from build123d import *

# Parameters (mm, degrees)
F2_SIZE        = 0.5
F3_SIZE        = 0.5
F4_SIZE2       = 1.3397459622
F4_SIZE        = 5
F6_D           = 7
F7_D           = 7
F7_CBORE_D     = 11
F7_CBORE_DEPTH = 7.5
F9_D           = 6
F9_DEPTH       = 5
F9_TIP         = 1.8025818571


with BuildPart() as f1:
    # F0 (on Front) → F1 (revolve)
    with BuildSketch(Plane.XZ):
        Polygon((0, 32), (0, 0), (66, 0), (66, 6), (54.15, 6), (54.15, 32), align=None)
    revolve(axis=Axis((0, 0, 31.825657934), (0, 0, 1)))

    # F2
    f2_edges = [f1.edges().sort_by_distance(p)[0] for p in [
        (-66, 0, 6),
    ]]
    chamfer(f2_edges, length=F2_SIZE)

    # F3
    f3_edges = [f1.edges().sort_by_distance(p)[0] for p in [
        (-66, 0, 0),
    ]]
    chamfer(f3_edges, length=F3_SIZE)

    # F4
    f4_edges = [f1.edges().sort_by_distance(p)[0] for p in [
        (-54.15, 0, 32),
    ]]
    chamfer(f4_edges, length=F4_SIZE, length2=F4_SIZE2)

    # F6 (through all)
    with Locations(Plane.XY.offset(32)):
        with Locations((-9, 0), (9, 0)):
            Hole(F6_D / 2)

    # F7 (through all)
    with Locations(Plane.XY.offset(32)):
        with Locations((9, 0), (-9, 0)):
            CounterBoreHole(F7_D / 2, F7_CBORE_D / 2, F7_CBORE_DEPTH)

    # F9
    with Locations(Plane(origin=(0, 0, 0), x_dir=(1, 0, 0), z_dir=(0, 0, -1))):
        with Locations((0, 0)):
            Hole(F9_D / 2, depth=F9_DEPTH)
            with Locations((0, 0, -(F9_DEPTH + F9_TIP / 2))):  # 118° drill point
                Cone(0, F9_D / 2, F9_TIP, mode=Mode.SUBTRACT)


solid = f1.part
Here's how the part is built. I have some questions about the finished solid (model axes, mm). A direction names the side the tool comes from. Round coordinates to 2 decimals unless told otherwise and drop trailing zeros. Order: outer loops, then holes, each group sorted by start corner. A loop starts at its lowest first (then second) coordinate and runs counter-clockwise, first axis right, second up. Notation, with made-up numbers: (18, 32.5) -> (70, 32.5) arc R21 ccw to (70, 43.5) -> close; hole circle Ø3 at (37.5, 54). An arc over 180 degrees is marked (long way). Use CSV: the item, a comma, the result in double quotes.
1. Thinking about a two-plate mould opening in Y: for faces 1 (the face through (-25, 49, 6)), 2 (the face through (-11.462, -51.618, 31.757)), 3 (the face through (-5, 0, 24.5)), which applies, pulls with the +Y half, pulls with the -Y half, needs draft (parallel to the pull), parting line crosses it, or undercut?
Recorded:
face 1,"needs draft"
face 2,"parting line crosses it"
face 3,"undercut"
2. I'm going to push flat-ended pins straight in: P1, Ø4, axis at y = 3, z = 17, coming from the -X side; P2, Ø3, axis at x = -16.5, z = 27, coming from the +Y side; P3, Ø1.5, axis at x = -2.5, z = 10, coming from the +Y side; P4, Ø9, axis at x = 9, y = 0, coming from the -Z side. Where does each tip first touch, or does it pass through?
Recorded:
P1,"stops at x = -54.14"
P2,"stops at y = 52.03"
P3,"stops at y = 54.12"
P4,"stops at z = 0"
3. I need wall thicknesses on line 1 along Y through (x, z) = (0, 3); line 2 along Y through (x, z) = (-9, 29.5); line 3 along X through (y, z) = (-2, 2). Which ranges of each line are inside material? Lowest first, please.
Recorded:
line 1,"y = -66 to -3, 3 to 66"
line 2,"y = -52.72 to -5.5, 5.5 to 52.72"
line 3,"x = -65.97 to -11.87, -6.13 to -2.24, 2.24 to 6.13, 11.87 to 65.97"
4. Which directions (+Z, -Z, +X, -X, +Y, -Y) give clear straight access to the entire face, cutting with the end or side of a thin tool? Please do faces 4 (the face through (14.08, -2.11, 28.3)), 5 (the face through (3, 0, 3)), 6 (the face through (60.967, -25.278, 3.035)).
Recorded:
face 4,"+Z"
face 5,"-Z"
face 6,"+Z, -Z"
5. I want a section at A-A on z = 29. List the corners of the cut face in (x, y) for me.
Recorded:
outline,"circle Ø107.23 at (0, 0); hole circle Ø11 at (-9, 0); hole circle Ø11 at (9, 0)"
6. I want a section at B-B on z = 19. List the corners of the cut face in (x, y) for me, and give its area (3 significant figures).
Recorded:
outline,"circle Ø108.3 at (0, 0); hole circle Ø7 at (-9, 0); hole circle Ø7 at (9, 0)"
area,"9,130 mm2"
